from build123d import *

# Parameters (mm, degrees)
F0_W     = 203.2
F0_H     = 25.4
F1_DEPTH = 25.4
F2_W     = 22.225
F2_H     = 22.2123
F3_DEPTH = 203.2
F5_R     = 2.5527
F6_DEPTH = 50.8
F7_D     = 5.1054


with BuildPart() as f1:
    # F0 (on Top) → F1 (new body)
    with BuildSketch(Plane.XY):
        with Locations((-7.462719, 18.38669)):
            Rectangle(F0_W, F0_H)
    extrude(amount=F1_DEPTH)

    # F2 (on face) → F3 (cut)
    with BuildSketch(Plane.YZ.offset(94.137281)):
        with Locations((18.38669, 12.70635)):
            Rectangle(F2_W, F2_H)
    extrude(amount=-F3_DEPTH, mode=Mode.SUBTRACT)

    # F5 (on face) → F6 (cut)
    with BuildSketch(Plane(origin=(0, 31.08669, 0), x_dir=(-1, 0, 0), z_dir=(0, 1, 0))):
        with Locations((-5.237281, 12.7)):
            Circle(F5_R)
        with Locations((-30.637281, 12.7)):
            Circle(F5_R)
        with Locations((20.162719, 12.7)):
            Circle(F5_R)
        with Locations((45.562719, 12.7)):
            Circle(F5_R)
        with Locations((70.962719, 12.7)):
            Circle(F5_R)
        with Locations((96.362719, 12.7)):
            Circle(F5_R)
        with Locations((-81.437281, 12.7)):
            Circle(F5_R)
        with Locations((-56.037281, 12.7)):
            Circle(F5_R)
    extrude(amount=-F6_DEPTH, mode=Mode.SUBTRACT)

    # F7 (through all)
    with Locations(Plane.XY.offset(25.4)):
        with Locations((81.437281, -7.01331), (-96.362719, 18.38669), (-70.962719, 18.38669), (30.637281, 18.38669), (-96.362719, -7.01331), (-20.162719, 18.38669), (81.437281, 18.38669), (-45.562719, -7.01331), (5.237281, -7.01331), (56.037281, -7.01331), (30.637281, -7.01331), (56.037281, 18.38669), (-45.562719, 18.38669), (-70.962719, -7.01331), (-20.162719, -7.01331), (5.237281, 18.38669)):
            Hole(F7_D / 2)


solid = f1.part
CAD build for the part. Positions are in the model's coordinates, mm. A direction names the side the tool comes from. Give positions to 0.01 mm unless a question says otherwise; leave off trailing zeros. Loops run counter-clockwise (first coordinate to the right, second up) from the corner with the lowest first, then second, coordinate; pieces in that order, holes last. Notation, with made-up numbers: M -6.75,23.25 L 4.25,23.25 A23 cw 4.25,31.25 Z; hole C 69,73.5 d2. An arc over 180 degrees is marked long. One line per question, with ' | ' between items. Start each with the question number.
1. Probe L1, parallel to Z at x = 71.5, y = 12.25; L2, parallel to Y at x = -50, z = 11. List the from-to ranges inside material, lowest first. Write a range as from..to.
2. Saw through at A-A on y = 26. Give the cut face in (x, z), plus the area to 3 significant figures.
3. Saw through at D-D on z = 12.7. State how many separate pieces and enclosed holes the cut face has, plus the area to 3 significant figures.
4. Two-plate mould, pull along X, no slides. Class faces 3 (the face through (-93.812, 18.499, 0.789)), 4 (the face through (-9, 5.687, 13)): pulls with the +X half, pulls with the -X half, needs draft (parallel to the pull), parting line crosses it, or undercut.
5. Flat gauge pin, fed straight in: pin 1 (4 mm diameter, centred on x = 56.04, z = 12.7, fed in from -Y). Where does the tip first touch, or does it go through?
6. 3-axis set-ups, long thin cutter, end or side, ignore diameter. For faces 1 (the face through (58.063, 30.304, 11.147)), 2 (the face through (-6, 29.499, 13)): which of +Z, -Z, +X, -X, +Y, -Y reach the whole face in a straight line?
7. Saw through at B-B on z = 3.5. Give the cut face in (x, y).
8. Saw through at C-C on x = -71. Give the cut face in (y, z), plus the area to 3 significant figures.
Result sheet:
1) L1: z = 0..1.6, 23.81..25.4 | L2: y = 5.69..7.27, 29.5..31.09
2) outline: M -109.06,0 L 94.14,0 L 94.14,1.6 L -109.06,1.6 Z; M -109.06,23.81 L 94.14,23.81 L 94.14,25.4 L -109.06,25.4 Z | area: 648 mm^2
3) separate pieces: 18 | enclosed holes: 0 | area: 515 mm^2
4) face 3: undercut | face 4: needs draft
5) pin 1: passes through
6) face 1: +Y, -Y | face 2: +X, -X
7) outline: M -109.06,5.69 L 94.14,5.69 L 94.14,7.27 L -109.06,7.27 Z; M -109.06,29.5 L 94.14,29.5 L 94.14,31.09 L -109.06,31.09 Z
8) outline: M 5.69,0 L 15.83,0 L 15.83,1.6 L 7.27,1.6 L 7.27,10.15 L 5.69,10.15 Z; M 5.69,15.25 L 7.27,15.25 L 7.27,23.81 L 15.83,23.81 L 15.83,25.4 L 5.69,25.4 Z; M 20.94,0 L 31.09,0 L 31.09,10.15 L 29.5,10.15 L 29.5,1.6 L 20.94,1.6 Z; M 20.94,23.81 L 29.5,23.81 L 29.5,15.25 L 31.09,15.25 L 31.09,25.4 L 20.94,25.4 Z | area: 119 mm^2
